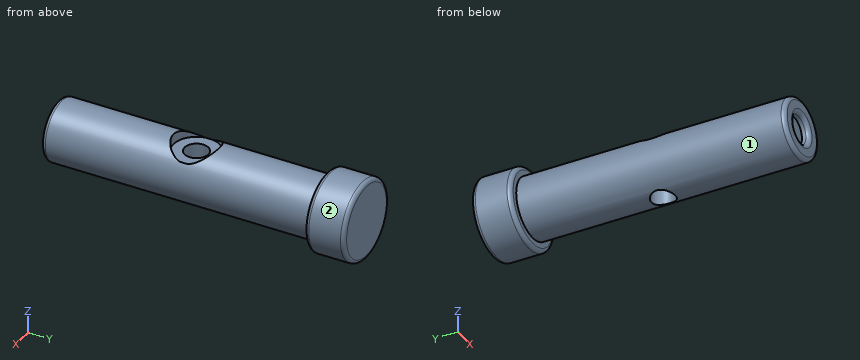
from build123d import *

# Parameters (mm, degrees)
VERRUNDUNG1_R                        = 0.5
SCHNITT_LINEAR_AUSTRAGEN1_DEPTH      = 40.635842378
SCHNITT_LINEAR_AUSTRAGEN1_DEPTH_BACK = 40.635842378
SKIZZE2_R                            = 1.5
SKIZZE3_R                            = 2.9
SCHNITT_LINEAR_AUSTRAGEN10_DEPTH     = 41.028115132


with BuildPart() as part:
    # Skizze1 → Rotation1 (revolve)
    with BuildSketch(Plane.XY):
        Polygon((0, 0), (0, -38), (-1.8, -38), (-1.8, -39), (-3.8, -39), (-3.8, -5), (-5, -5), (-5, 0), align=None)
    revolve(axis=Axis((0, 0, 0), (0, -1, 0)))

    # Verrundung1
    verrundung1_edges = [part.edges().sort_by_distance(p)[0] for p in [
        (5, 0, 0),
        (5, -5, 0),
        (3.8, -39, 0),
        (1.8, -39, 0),
    ]]
    fillet(verrundung1_edges, radius=VERRUNDUNG1_R)

    # Skizze2 → Schnitt-Linear austragen1 (cut, two sides: drawn at the far end of the back side and taken through both)
    with BuildSketch(Plane.XY.offset(-SCHNITT_LINEAR_AUSTRAGEN1_DEPTH_BACK)):
        with Locations((0, -21.5)):
            Circle(SKIZZE2_R)
    extrude(amount=SCHNITT_LINEAR_AUSTRAGEN1_DEPTH + SCHNITT_LINEAR_AUSTRAGEN1_DEPTH_BACK, mode=Mode.SUBTRACT)

    # Skizze3 → Schnitt-Linear austragen10 (cut, through all)
    with BuildSketch(Plane.XY.offset(2.5)):
        with Locations((0, -21.5)):
            Circle(SKIZZE3_R)
    extrude(amount=SCHNITT_LINEAR_AUSTRAGEN10_DEPTH, mode=Mode.SUBTRACT)


solid = part.part
Build history of the part. All positions in model axes, mm. Face numbers are marked on the shaded views. A direction names the side the tool comes from. Coordinates: 2 decimals unless noted, no trailing zeros. Write each loop counter-clockwise with the first axis right and the second up, starting at its lowest first coordinate (ties: lowest second). Pieces come first, ordered by that corner, then holes. Notation, with made-up numbers: (72.5, 3) -> (100.5, 3) arc R15 cw to (100.5, 15) -> close; hole circle Ø1 at (20.25, -18). An arc over 180 degrees is marked (long way). Use CSV: the item, a comma, the result in double quotes. Start each with the question number.
Q1. Cut at C-C, the plane y = -16.5. List the corners of the cut face in (x, z).
Q2. Cut at B-B, the plane y = -21.5. List the corners of the cut face in (x, z).
Q3. Flat gauge pins, fed straight in: pin 1 Ø1 at (y, z) = (-18.5, -3) entering from +X; pin 2 Ø6 at (y, z) = (-29.5, -0.5) entering from -X; pin 3 Ø1.5 at (y, z) = (-32, -2.5) entering from +X. Where does each tip first touch, or does it go through?
Q4. 3-axis set-ups, long thin cutter, end or side, ignore diameter. For the marked faces 1 and 2: which of +Z, -Z, +X, -X, +Y, -Y reach the whole face in a straight line?
Q5. Cut at A-A, the plane x = 0. List the corners of the cut face in (y, z), then the cut area to 3 significant figures.
Q6. Drill centre lines: probe 1 along X at (y, z) = (-38.3, 0); probe 2 along X at (y, z) = (-21.5, -0.25). Where is each one in solid material? Low to high.
Checked values:
1,outline,"circle Ø7.6 at (0, 0)"
2,outline,"(-2.86, 2.5) arc R3.8 ccw to (-1.5, -3.49) -> (-1.5, 2.5) -> close; (1.5, -3.49) arc R3.8 ccw to (2.86, 2.5) -> (1.5, 2.5) -> close"
3,pin 1,"stops at x = 2.86"
3,pin 2,"stops at x = -3.8"
3,pin 3,"stops at x = 3.37"
4,face 1,"-Y"
4,face 2,"+Y, -Y"
5,outline,"(-39, -3.3) arc R0.5 ccw to (-38.5, -3.8) -> (-23, -3.8) -> (-23, 2.5) -> (-24.4, 2.5) -> (-24.4, 3.8) -> (-38.5, 3.8) arc R0.5 ccw to (-39, 3.3) -> (-39, 2.3) arc R0.5 ccw to (-38.5, 1.8) -> (-38, 1.8) -> (-38, -1.8) -> (-38.5, -1.8) arc R0.5 ccw to (-39, -2.3) -> close; (-20, -3.8) -> (-5, -3.8) -> (-5, -4.5) arc R0.5 ccw to (-4.5, -5) -> (-0.5, -5) arc R0.5 ccw to (0, -4.5) -> (0, 4.5) arc R0.5 ccw to (-0.5, 5) -> (-4.5, 5) arc R0.5 ccw to (-5, 4.5) -> (-5, 3.8) -> (-18.6, 3.8) -> (-18.6, 2.5) -> (-20, 2.5) -> close"
5,area,"278 mm²"
6,probe 1,"x = -3.8 to -1.8, 1.8 to 3.8"
6,probe 2,"x = -3.79 to -1.5, 1.5 to 3.79"
